Part model, mm, in its own coordinate system. A direction names the side the tool comes from. Coordinates: 2 decimals unless noted, no trailing zeros. Loops run counter-clockwise (first coordinate to the right, second up) from the corner with the lowest first, then second, coordinate; pieces in that order, holes last. Notation, with made-up numbers: (-12, 86) -> (-2, 86) arc R3 cw to (-2, 90) -> close; hole circle Ø6 at (-0.5, 53). An arc over 180 degrees is marked (long way). Use one line per item in the form item = value. Start each with the question number.
(1) Drill centre lines: L1, parallel to X at y = -10, z = 7.25; L2, parallel to Y at x = 6, z = 2.35; L3, parallel to Z at x = 19.5, y = -24. Where is each one in solid material? Low to high. Write a range as [from, to].
(2) Pin check, flat tips, straight feed: P1, Ø1.5, axis at x = 6.5, z = 2, coming from the -Y side; P2, Ø1.8, axis at x = 3.5, y = -2.5, coming from the +Z side; P3, Ø5, axis at x = 8.5, z = 4, coming from the +Y side. Stop position of each tip, or through.
(3) Band-saw the part on C-C on z = 4.5. Give the cut face in (x, y), then the cut area to 3 significant figures.
(4) Band-saw the part on D-D on y = -11.5. Give the cut face in (x, z), then the cut area to 3 significant figures.
(5) Band-saw the part on B-B on x = 6. Give the cut face in (y, z).
(6) Mould opens along Y. For faces 1 (the flat face through (19, -19, 4)), 2 (the flat face through (24, -9, 5)), 3 (the flat face through (13, 0, 2)), 4 (the flat face through (19, -25.6, 3)) say: +Y half, -Y half, draft (parallel to the pull), parting line (faces both ways), or undercut.
(7) Band-saw the part on A-A on z = 2. Give the cut face in (x, y).
(8) 3-axis set-ups, long thin cutter, end or side, ignore diameter. For faces 5 (the flat face through (4, -3, 5)), 6 (the flat face through (13, -9, 5)), 7 (the flat face through (22, -10, 6)): which of +Z, -Z, +X, -X, +Y, -Y reach the whole face in a straight line?
```python
from build123d import *

# Parameters (mm, degrees)
SKETCH_1_W          = 26
SKETCH_1_H          = 6
SKETCH_1_R          = 1.5
EXTRUDE_1_DEPTH     = 5
SKETCH_2_W          = 4
SKETCH_2_H          = 32.6
EXTRUDE_2_DEPTH     = 3.8
SKETCH_3_W          = 6.5
SKETCH_3_H          = 6.5
CUT_EXTRUDE_1_DEPTH = 1
SKETCH_4_W          = 14.5
SKETCH_4_H          = 12.6
EXTRUDE_3_DEPTH     = 5
SKETCH_5_W          = 6.5
SKETCH_5_H          = 12.6
CUT_EXTRUDE_2_DEPTH = 1


with BuildPart() as part:
    # 草图1 → 凸台-拉伸1 (new body)
    with BuildSketch(Plane.XY):
        with Locations((13, -3)):
            Rectangle(SKETCH_1_W, SKETCH_1_H)
        with Locations((6, -3)):
            Circle(SKETCH_1_R, mode=Mode.SUBTRACT)
    extrude(amount=EXTRUDE_1_DEPTH)

    # 草图2 → 凸台-拉伸2 (add)
    with BuildSketch(Plane.XY.offset(5)):
        with Locations((24, -9.3)):
            Rectangle(SKETCH_2_W, SKETCH_2_H)
        with Locations((13.5, -9.3)):
            Rectangle(SKETCH_2_W, SKETCH_2_H)
    extrude(amount=EXTRUDE_2_DEPTH)

    # 草图3 → 切除-拉伸1 (cut)
    with BuildSketch(Plane.XY.offset(5)):
        with Locations((18.75, -2.75)):
            Rectangle(SKETCH_3_W, SKETCH_3_H)
    extrude(amount=-CUT_EXTRUDE_1_DEPTH, mode=Mode.SUBTRACT)

    # 草图4 → 凸台-拉伸3 (add)
    with BuildSketch(Plane(origin=(0, 0, 5), x_dir=(-1, 0, 0), z_dir=(0, 0, -1))):
        with Locations((-18.75, -19.3)):
            Rectangle(SKETCH_4_W, SKETCH_4_H)
    extrude(amount=EXTRUDE_3_DEPTH)

    # 草图5 → 切除-拉伸2 (cut)
    with BuildSketch(Plane.XY.offset(5)):
        with Locations((18.75, -19.3)):
            Rectangle(SKETCH_5_W, SKETCH_5_H)
    extrude(amount=-CUT_EXTRUDE_2_DEPTH, mode=Mode.SUBTRACT)


solid = part.part
```
A:
q1.L1 = [11.5, 15.5], [22, 26]
q1.L2 = [-6, -4.5], [-1.5, 0]
q1.L3 = [0, 4]
q2.P1 = -6
q2.P2 = 5
q2.P3 = 0
q3.outline = (0, -6) -> (15.5, -6) -> (15.5, 0) -> (0, 0) -> close; (11.5, -25.6) -> (15.5, -25.6) -> (15.5, -13) -> (11.5, -13) -> close; (22, -25.6) -> (26, -25.6) -> (26, -13) -> (22, -13) -> close; (22, -6) -> (26, -6) -> (26, 0) -> (22, 0) -> close; hole circle Ø3 at (6, -3)
q3.area = 211 mm²
q4.outline = (11.5, 5) -> (15.5, 5) -> (15.5, 8.8) -> (11.5, 8.8) -> close; (22, 5) -> (26, 5) -> (26, 8.8) -> (22, 8.8) -> close
q4.area = 30.4 mm²
q5.outline = (-6, 0) -> (-4.5, 0) -> (-4.5, 5) -> (-6, 5) -> close; (-1.5, 0) -> (0, 0) -> (0, 5) -> (-1.5, 5) -> close
q6.face_1 = draft
q6.face_2 = undercut
q6.face_3 = +Y half
q6.face_4 = -Y half
q7.outline = (0, -6) -> (26, -6) -> (26, 0) -> (0, 0) -> close; (11.5, -25.6) -> (26, -25.6) -> (26, -13) -> (11.5, -13) -> close; hole circle Ø3 at (6, -3)
q8.face_5 = +Z, -X, +Y, -Y
q8.face_6 = -Z, +X, -X
q8.face_7 = +Z, +Y, -Y
